```python
from build123d import *

# Parameters (mm, degrees)
EXTRUDE_1_DEPTH      = 45.4
SKETCH_2_W           = 25
SKETCH_2_H           = 6.5
CUT_EXTRUDE_1_DEPTH  = 0.5
SKETCH_3_W           = 6.5
SKETCH_3_H           = 1.414213562
CUT_EXTRUDE_2_DEPTH  = 0.5
SKETCH_4_W           = 6.5
SKETCH_4_H           = 8
CUT_EXTRUDE_3_DEPTH  = 0.5
SKETCH_5_W           = 6.5
SKETCH_5_H           = 1.414213562
CUT_EXTRUDE_4_DEPTH  = 0.5
SKETCH_6_W           = 6.4
SKETCH_6_H           = 6.5
CUT_EXTRUDE_5_DEPTH  = 0.5
SKETCH_7_W           = 6.5
SKETCH_7_H           = 1.414213563
CUT_EXTRUDE_6_DEPTH  = 0.5
SKETCH_8_W           = 6.5
SKETCH_8_H           = 8
CUT_EXTRUDE_7_DEPTH  = 0.5
SKETCH_9_W           = 6.5
SKETCH_9_H           = 1.414213562
CUT_EXTRUDE_8_DEPTH  = 0.5
SKETCH_10_W          = 6.4
SKETCH_10_H          = 6.5
CUT_EXTRUDE_9_DEPTH  = 0.5
SKETCH_11_W          = 25
SKETCH_11_H          = 6.5
CUT_EXTRUDE_10_DEPTH = 0.5
SKETCH_12_W          = 6.5
SKETCH_12_H          = 1.414213563
CUT_EXTRUDE_11_DEPTH = 0.5
SKETCH_13_W          = 6.5
SKETCH_13_H          = 8
CUT_EXTRUDE_12_DEPTH = 0.5
SKETCH_14_W          = 6.5
SKETCH_14_H          = 1.414213562
CUT_EXTRUDE_13_DEPTH = 0.5
SKETCH_15_W          = 6.4
SKETCH_15_H          = 6.5
CUT_EXTRUDE_14_DEPTH = 0.5
SKETCH_16_W          = 6.5
SKETCH_16_H          = 1.414213562
CUT_EXTRUDE_15_DEPTH = 0.5
SKETCH_17_W          = 6.5
SKETCH_17_H          = 8
CUT_EXTRUDE_16_DEPTH = 0.5
SKETCH_18_W          = 6.5
SKETCH_18_H          = 1.414213562
CUT_EXTRUDE_17_DEPTH = 0.5
SKETCH_19_W          = 6.4
SKETCH_19_H          = 6.5
CUT_EXTRUDE_18_DEPTH = 0.5
SKETCH_20_R          = 1.5
CUT_EXTRUDE_19_DEPTH = 3.5
SKETCH_21_R          = 1.5
CUT_EXTRUDE_21_DEPTH = 3.5
CUT_EXTRUDE_START    = -3.5
SKETCH_22_R          = 1.5
CUT_EXTRUDE_22_DEPTH = 3.5


with BuildPart() as part:
    # 草图1 → 凸台-拉伸1 (new body)
    with BuildSketch(Plane.XY):
        Polygon((-15.119558261, 17.576687619), (-3.69760958, 17.576687619), (-3.282491259, 16.686463507), (-4.740379733, 15.665639007), (-4.740379733, 15.378970272), (-3.30858392, 14.37641605), (-3.30858392, 12.576687619), (3.09141608, 12.576687619), (4.09141608, 13.576687619), (4.09141608, 21.576687619), (3.09141608, 22.576687619), (-21.90858392, 22.576687619), (-22.90858392, 21.576687619), (-22.90858392, 13.576687619), (-21.90858392, 12.576687619), (-15.50858392, 12.576687619), (-15.50858392, 14.37641605), (-14.076788108, 15.378970272), (-14.076788108, 15.665639007), (-15.534676582, 16.686463507), align=None)
    extrude(amount=EXTRUDE_1_DEPTH)

    # 草图2 → 切除-拉伸1 (cut)
    with BuildSketch(Plane(origin=(0, 22.576687619, 0), x_dir=(1, 0, 0), z_dir=(0, 1, 0))):
        with Locations((-9.40858392, -3.25)):
            Rectangle(SKETCH_2_W, SKETCH_2_H)
    extrude(amount=-CUT_EXTRUDE_1_DEPTH, mode=Mode.SUBTRACT)

    # 草图3 → 切除-拉伸2 (cut)
    with BuildSketch(Plane(origin=(-22.24263577, 22.24263577, 0), x_dir=(0, 0, 1), z_dir=(-0.7071067811865477, 0.7071067811865475, 0))):
        with Locations((3.25, -0.234686125)):
            Rectangle(SKETCH_3_W, SKETCH_3_H)
    extrude(amount=-CUT_EXTRUDE_2_DEPTH, mode=Mode.SUBTRACT)

    # 草图4 → 切除-拉伸3 (cut)
    with BuildSketch(Plane.ZY.offset(22.90858392)):
        with Locations((3.25, 17.576687619)):
            Rectangle(SKETCH_4_W, SKETCH_4_H)
    extrude(amount=-CUT_EXTRUDE_3_DEPTH, mode=Mode.SUBTRACT)

    # 草图5 → 切除-拉伸4 (cut)
    with BuildSketch(Plane(origin=(-4.665948151, -4.665948151, 0), x_dir=(0, 0, 1), z_dir=(-0.7071067811865469, -0.7071067811865481, 0))):
        with Locations((3.25, 25.091876138)):
            Rectangle(SKETCH_5_W, SKETCH_5_H)
    extrude(amount=-CUT_EXTRUDE_4_DEPTH, mode=Mode.SUBTRACT)

    # 草图6 → 切除-拉伸5 (cut)
    with BuildSketch(Plane.XZ.offset(-12.576687619)):
        with Locations((-18.70858392, 3.25)):
            Rectangle(SKETCH_6_W, SKETCH_6_H)
    extrude(amount=-CUT_EXTRUDE_5_DEPTH, mode=Mode.SUBTRACT)

    # 草图7 → 切除-拉伸6 (cut)
    with BuildSketch(Plane(origin=(12.834051849, 12.834051849, 0), x_dir=(0, 0, -1), z_dir=(0.7071067811865478, 0.7071067811865472, 0))):
        with Locations((-3.25, 13.071060858)):
            Rectangle(SKETCH_7_W, SKETCH_7_H)
    extrude(amount=-CUT_EXTRUDE_6_DEPTH, mode=Mode.SUBTRACT)

    # 草图8 → 切除-拉伸7 (cut)
    with BuildSketch(Plane(origin=(4.09141608, 0, 0), x_dir=(0, 0, -1), z_dir=(1, 0, 0))):
        with Locations((-3.25, 17.576687619)):
            Rectangle(SKETCH_8_W, SKETCH_8_H)
    extrude(amount=-CUT_EXTRUDE_7_DEPTH, mode=Mode.SUBTRACT)

    # 草图9 → 切除-拉伸8 (cut)
    with BuildSketch(Plane(origin=(-4.74263577, 4.74263577, 0), x_dir=(0, 0, -1), z_dir=(0.7071067811865472, -0.7071067811865478, 0))):
        with Locations((-3.25, 11.786129155)):
            Rectangle(SKETCH_9_W, SKETCH_9_H)
    extrude(amount=-CUT_EXTRUDE_8_DEPTH, mode=Mode.SUBTRACT)

    # 草图10 → 切除-拉伸9 (cut)
    with BuildSketch(Plane.XZ.offset(-12.576687619)):
        with Locations((-0.10858392, 3.25)):
            Rectangle(SKETCH_10_W, SKETCH_10_H)
    extrude(amount=-CUT_EXTRUDE_9_DEPTH, mode=Mode.SUBTRACT)

    # 草图11 → 切除-拉伸10 (cut)
    with BuildSketch(Plane(origin=(0, 22.576687619, 0), x_dir=(1, 0, 0), z_dir=(0, 1, 0))):
        with Locations((-9.40858392, -42.15)):
            Rectangle(SKETCH_11_W, SKETCH_11_H)
    extrude(amount=-CUT_EXTRUDE_10_DEPTH, mode=Mode.SUBTRACT)

    # 草图12 → 切除-拉伸11 (cut)
    with BuildSketch(Plane(origin=(12.834051849, 12.834051849, 0), x_dir=(0, 0, -1), z_dir=(0.7071067811865478, 0.7071067811865472, 0))):
        with Locations((-42.15, 13.071060858)):
            Rectangle(SKETCH_12_W, SKETCH_12_H)
    extrude(amount=-CUT_EXTRUDE_11_DEPTH, mode=Mode.SUBTRACT)

    # 草图13 → 切除-拉伸12 (cut)
    with BuildSketch(Plane(origin=(4.09141608, 0, 0), x_dir=(0, 0, -1), z_dir=(1, 0, 0))):
        with Locations((-42.15, 17.576687619)):
            Rectangle(SKETCH_13_W, SKETCH_13_H)
    extrude(amount=-CUT_EXTRUDE_12_DEPTH, mode=Mode.SUBTRACT)

    # 草图14 → 切除-拉伸13 (cut)
    with BuildSketch(Plane(origin=(-4.74263577, 4.74263577, 0), x_dir=(0, 0, -1), z_dir=(0.7071067811865472, -0.7071067811865478, 0))):
        with Locations((-42.15, 11.786129155)):
            Rectangle(SKETCH_14_W, SKETCH_14_H)
    extrude(amount=-CUT_EXTRUDE_13_DEPTH, mode=Mode.SUBTRACT)

    # 草图15 → 切除-拉伸14 (cut)
    with BuildSketch(Plane.XZ.offset(-12.576687619)):
        with Locations((-0.10858392, 42.15)):
            Rectangle(SKETCH_15_W, SKETCH_15_H)
    extrude(amount=-CUT_EXTRUDE_14_DEPTH, mode=Mode.SUBTRACT)

    # 草图16 → 切除-拉伸15 (cut)
    with BuildSketch(Plane(origin=(-22.24263577, 22.24263577, 0), x_dir=(0, 0, 1), z_dir=(-0.7071067811865477, 0.7071067811865475, 0))):
        with Locations((42.15, -0.234686125)):
            Rectangle(SKETCH_16_W, SKETCH_16_H)
    extrude(amount=-CUT_EXTRUDE_15_DEPTH, mode=Mode.SUBTRACT)

    # 草图17 → 切除-拉伸16 (cut)
    with BuildSketch(Plane.ZY.offset(22.90858392)):
        with Locations((42.15, 17.576687619)):
            Rectangle(SKETCH_17_W, SKETCH_17_H)
    extrude(amount=-CUT_EXTRUDE_16_DEPTH, mode=Mode.SUBTRACT)

    # 草图18 → 切除-拉伸17 (cut)
    with BuildSketch(Plane(origin=(-4.665948151, -4.665948151, 0), x_dir=(0, 0, 1), z_dir=(-0.7071067811865469, -0.7071067811865481, 0))):
        with Locations((42.15, 25.091876138)):
            Rectangle(SKETCH_18_W, SKETCH_18_H)
    extrude(amount=-CUT_EXTRUDE_17_DEPTH, mode=Mode.SUBTRACT)

    # 草图19 → 切除-拉伸18 (cut)
    with BuildSketch(Plane.XZ.offset(-12.576687619)):
        with Locations((-18.70858392, 42.15)):
            Rectangle(SKETCH_19_W, SKETCH_19_H)
    extrude(amount=-CUT_EXTRUDE_18_DEPTH, mode=Mode.SUBTRACT)

    # 草图20 → 切除-拉伸19 (cut)
    with BuildSketch(Plane(origin=(0, 22.576687619, 0), x_dir=(1, 0, 0), z_dir=(0, 1, 0))):
        with Locations(Location((-19.40858392, -12.7, 0), (0, 0, 270))):
            Circle(SKETCH_20_R)
        with Locations(Location((0.59141608, -12.7, 0), (0, 0, 270))):
            Circle(SKETCH_20_R)
        with Locations(Location((0.59141608, -32.7, 0), (0, 0, 270))):
            Circle(SKETCH_20_R)
        with Locations(Location((-19.40858392, -32.7, 0), (0, 0, 270))):
            Circle(SKETCH_20_R)
    extrude(amount=-CUT_EXTRUDE_19_DEPTH, mode=Mode.SUBTRACT)

    # 草图21 → 切除-拉伸21 (cut)
    with BuildSketch(Plane.XY.offset(45.4)):
        with Locations((-16.40858392, 19.576687619)):
            Circle(SKETCH_21_R)
        with Locations((-2.40858392, 19.576687619)):
            Circle(SKETCH_21_R)
    extrude(amount=-CUT_EXTRUDE_21_DEPTH, mode=Mode.SUBTRACT)

    # 草图22 → 切除-拉伸22 (cut)
    with BuildSketch(Plane(origin=(0, 0, 0), x_dir=(-1, 0, 0), z_dir=(0, 0, -1)).offset(CUT_EXTRUDE_START)):
        with Locations(Location((2.40858392, 19.576687619, 0), (0, 0, 180))):
            Circle(SKETCH_22_R)
        with Locations(Location((16.40858392, 19.576687619, 0), (0, 0, 180))):
            Circle(SKETCH_22_R)
    extrude(amount=CUT_EXTRUDE_22_DEPTH, mode=Mode.SUBTRACT)


solid = part.part
```
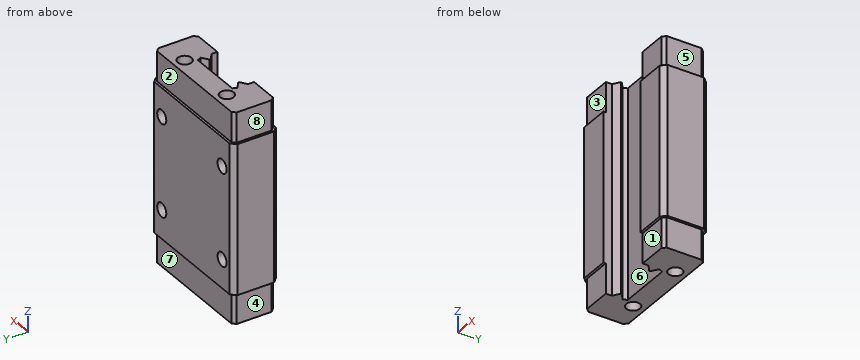
Verification items for the finished model (mm, model axes). Face numbers are marked on the shaded views. A direction names the side the tool comes from. Give positions to 0.01 mm unless a question says otherwise; leave off trailing zeros. Loops run counter-clockwise (first coordinate to the right, second up) from the corner with the lowest first, then second, coordinate; pieces in that order, holes last.
1. Section check D-D, the plane z = 32.7. Enter the section's corners in (x, y).
2. Section check A-A, the plane z = 5.5. Enter the section's corners in (x, y), then the cut area to 3 significant figures.
3. Go/stop test with flat-tipped pins: pin 1 Ø0.9 at (x, z) = (-20, 13) entering from +Y; pin 2 Ø5 at (x, z) = (-1.5, 43.5) entering from -Y; pin 3 Ø2.5 at (x, y) = (-2.41, 19.58) entering from +Z. Record where each tip stops, or that it passes through.
4. Thickness scan on line 1 (Z direction, x = 0.75, y = 22); line 2 (X direction, y = 16.75, z = 16.5); line 3 (Z direction, x = -20.5, y = 20). Record the ranges inside material, lowest first.
5. Mould release check, pull along X, two halves, no side actions. Record for the marked faces 6, 7 and 8: released by +X, released by -X, zero draft, split by the parting line, or undercut.
6. Section check C-C, the plane z = 26.5. Enter the section's corners in (x, y), then the cut area to 3 significant figures.
7. Section check B-B, the plane x = -13. Enter the section's corners in (y, z).
8. Set-up check for the marked faces 1, 2, 3, 4 and 5: record each of +Z, -Z, +X, -X, +Y, -Y from which the full face is reachable in a straight line by a thin tool's end or side.
Geometry says:
1. outline: (-22.91, 13.58) - (-21.91, 12.58) - (-15.51, 12.58) - (-15.51, 14.38) - (-14.08, 15.38) - (-14.08, 15.67) - (-15.53, 16.69) - (-15.12, 17.58) - (-3.7, 17.58) - (-3.28, 16.69) - (-4.74, 15.67) - (-4.74, 15.38) - (-3.31, 14.38) - (-3.31, 12.58) - (3.09, 12.58) - (4.09, 13.58) - (4.09, 21.58) - (3.09, 22.58) - (2.09, 22.58) - (2.09, 19.08) - (-0.91, 19.08) - (-0.91, 22.58) - (-17.91, 22.58) - (-17.91, 19.08) - (-20.91, 19.08) - (-20.91, 22.58) - (-21.91, 22.58) - (-22.91, 21.58) - close
2. outline: (-22.41, 13.78) - (-21.7, 13.08) - (-15.51, 13.08) - (-15.51, 14.38) - (-14.08, 15.38) - (-14.08, 15.67) - (-15.53, 16.69) - (-15.12, 17.58) - (-3.7, 17.58) - (-3.28, 16.69) - (-4.74, 15.67) - (-4.74, 15.38) - (-3.31, 14.38) - (-3.31, 13.08) - (2.88, 13.08) - (3.59, 13.78) - (3.59, 21.37) - (2.88, 22.08) - (-21.7, 22.08) - (-22.41, 21.37) - close
2. area: 182 mm2
3. pin 1: stops at y = 19.08
3. pin 2: stops at y = 13.08
3. pin 3: stops at z = 41.9
4. line 1: z = 0 to 11.21, 14.19 to 31.21, 34.19 to 45.4
4. line 2: x = -22.91 to -15.51, -3.31 to 4.09
4. line 3: z = 0 to 11.67, 13.73 to 31.67, 33.73 to 45.4
5. face 6: undercut
5. face 7: zero draft
5. face 8: released by -X
6. outline: (-22.91, 13.58) - (-21.91, 12.58) - (-15.51, 12.58) - (-15.51, 14.38) - (-14.08, 15.38) - (-14.08, 15.67) - (-15.53, 16.69) - (-15.12, 17.58) - (-3.7, 17.58) - (-3.28, 16.69) - (-4.74, 15.67) - (-4.74, 15.38) - (-3.31, 14.38) - (-3.31, 12.58) - (3.09, 12.58) - (4.09, 13.58) - (4.09, 21.58) - (3.09, 22.58) - (-21.91, 22.58) - (-22.91, 21.58) - close
6. area: 211 mm2
7. outline: (17.58, 0) - (22.08, 0) - (22.08, 6.5) - (22.58, 6.5) - (22.58, 38.9) - (22.08, 38.9) - (22.08, 45.4) - (17.58, 45.4) - close
8. face 1: -Z, +X, -X, -Y
8. face 2: +Z, +X, -X, +Y
8. face 3: +Z, +X, -X, -Y
8. face 4: -Z, -X, +Y, -Y
8. face 5: +Z, +X, +Y, -Y
